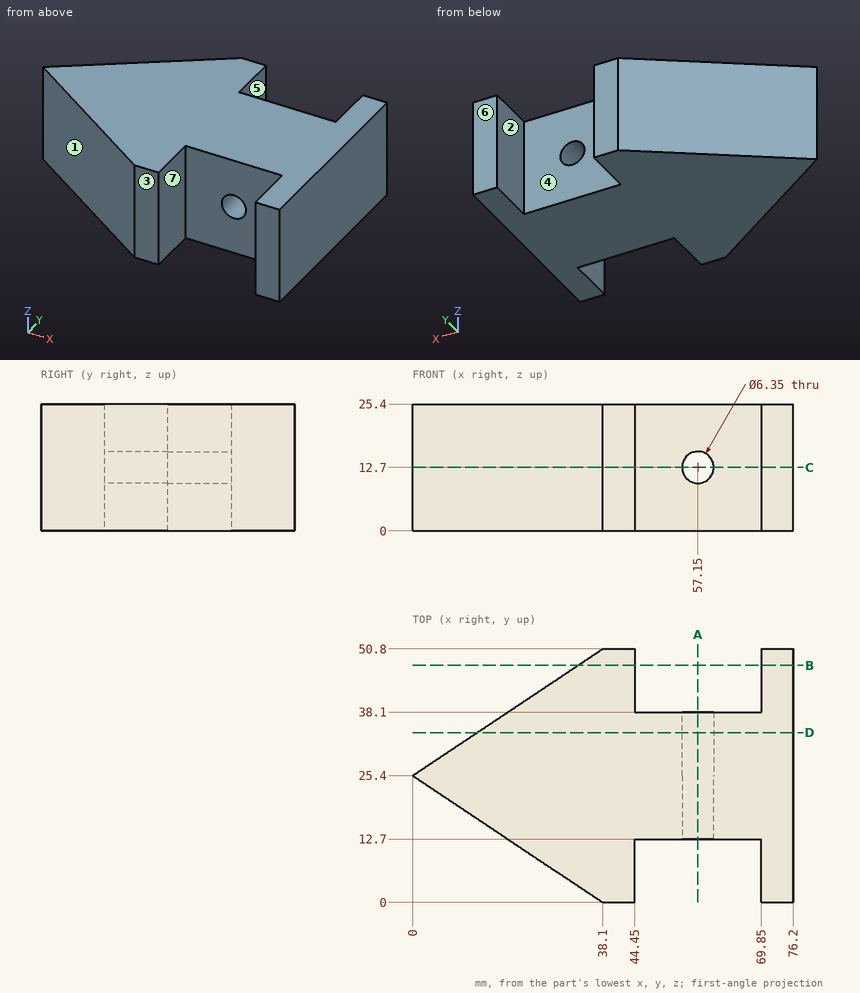
The drawing under review shows one solid part. Ordinate dimensions are in mm from its lowest x, y, z. A direction names the side the tool comes from. Give positions to 0.01 mm unless a question says otherwise; leave off trailing zeros. Order: outer loops, then holes, each group sorted by start corner. A loop starts at its lowest first (then second) coordinate and runs counter-clockwise, first axis right, second up. Notation, with made-up numbers: (36.25, 68.5) - (41.25, 68.5) arc R25 cw to (41.25, 84.5) - close; hole circle Ø7 at (74, 24). An arc over 180 degrees is marked (long way). Answer as a JSON object with one key per item and string values. Group by question number.
Item 1: Take a section at A-A on x = 57.15. Give the boundary of the cut face in (y, z) (3 decimals).
Item 2: Take a section at D-D on y = 34. Give the boundary of the cut face in (x, z) (3 decimals).
Item 3: Take a section at C-C on z = 12.7. Give the boundary of the cut face in (x, y) (3 decimals).
Item 4: Draft analysis for pull direction X (two halves, no side actions). For the marked faces 1, 2, 3 and 4, state which applies: pulls with the +X half, pulls with the -X half, needs draft (parallel to the pull), parting line crosses it, or undercut.
Item 5: Machinability: for the marked faces 5, 6 and 7, which of the approach directions +Z, -Z, +X, -X, +Y, -Y give a long, thin tool a straight path to every point of the face, cutting with its end or side? Answer none if there is none.
Item 6: Take a section at B-B on y = 47.5. Give the boundary of the cut face in (x, z), and give its area (3 significant figures).
Item 7: Clearance check with flat-ended pins moving along their axes: pin 1 Ø5 at (y, z) = (9, 11.5) entering from -X; pin 2 Ø7.5 at (x, z) = (57.15, 12.7) entering from +Y; pin 3 Ø10 at (y, z) = (4.5, 15.5) entering from -X; pin 4 Ø8 at (x, y) = (11, 12) entering from -Z. State where each tip first meets the part, or that it passes through.
Item 8: Wall thickness on line 1 along Z through (x, y) = (57, 29); line 2 along Y through (x, z) = (65, 20); line 3 along X through (y, z) = (48.5, 1): over which ranges is each line inside the solid? List them lowest first.
Reported:
{
 "1": {"outline": "(12.7, 0) - (38.1, 0) - (38.1, 9.525) - (12.7, 9.525) - close; (12.7, 15.875) - (38.1, 15.875) - (38.1, 25.4) - (12.7, 25.4) - close"},
 "2": {"outline": "(12.9, 0) - (76.2, 0) - (76.2, 25.4) - (12.9, 25.4) - close; hole circle Ø6.35 at (57.15, 12.7)"},
 "3": {"outline": "(0, 25.4) - (38.1, 0) - (44.45, 0) - (44.45, 12.7) - (53.975, 12.7) - (53.975, 38.1) - (44.45, 38.1) - (44.45, 50.8) - (38.1, 50.8) - close; (60.325, 12.7) - (69.85, 12.7) - (69.85, 0) - (76.2, 0) - (76.2, 50.8) - (69.85, 50.8) - (69.85, 38.1) - (60.325, 38.1) - close"},
 "4": {"face 1": "pulls with the -X half", "face 2": "undercut", "face 3": "needs draft", "face 4": "undercut"},
 "5": {"face 5": "+Z, -Z, +Y", "face 6": "+Z, -Z, +X, -X, +Y", "face 7": "+Z, -Z, -Y"},
 "6": {"outline": "(33.15, 0) - (44.45, 0) - (44.45, 25.4) - (33.15, 25.4) - close; (69.85, 0) - (76.2, 0) - (76.2, 25.4) - (69.85, 25.4) - close", "area": "448 mm^2"},
 "7": {"pin 1": "x = 20.85", "pin 2": "y = 38.1", "pin 3": "x = 23.85", "pin 4": "through"},
 "8": {"line 1": "0 to 9.53, 15.87 to 25.4", "line 2": "12.7 to 38.1", "line 3": "34.65 to 44.45, 69.85 to 76.2"}
}
